Can you work these out from the model? Positions are in its coordinate system, mm. A direction names the side the tool comes from. Round coordinates to 2 decimals unless told otherwise and drop trailing zeros. Loops run counter-clockwise (first coordinate to the right, second up) from the corner with the lowest first, then second, coordinate; pieces in that order, holes last. Notation, with made-up numbers: M 68,84.5 L 114,84.5 A16 ccw 114,92.5 Z; hole C 19.5,-29 d3. An arc over 180 degrees is marked long. Use a Markdown table: item, result. Add a question column.
```python
from build123d import *

# Parameters (mm, degrees)
F3_R        = 44
F3_W        = 60
F3_H        = 60
F4_DEPTH    = 13
F5_T1_DEPTH = 28


# Not quite as in the source:
# - a fillet or chamfer that OpenCascade refuses, or shapes differently, is made with other operations: its cross-section is extruded or revolved along the edge and cut away or added


with BuildPart() as f2:
    # F1 (on Front) → F2 (revolve)
    with BuildSketch(Plane.XZ):
        with BuildLine():
            Line((-18, 6), (0, 6))
            Line((0, 6), (7, 6))
            Line((7, 6), (7, 8))
            Line((7, 8), (9, 8))
            Line((9, 8), (9, 10.5))
            Line((9, 10.5), (19, 10.5))
            Line((19, 10.5), (19, 44))
            Line((19, 44), (6, 44))
            Line((6, 44), (6, 42))
            Line((6, 42), (0, 42))
            Line((0, 42), (0, 20))
            Line((0, 20), (-4, 20))
            ThreePointArc((-4, 20), (-10, 14), (-16, 20))
            Line((-16, 20), (-20, 20))
            Line((-20, 20), (-20, 18))
            Line((-20, 18), (-30, 18))
            Line((-30, 18), (-30, 10.5))
            Line((-30, 10.5), (-20, 10.5))
            Line((-20, 10.5), (-20, 8))
            Line((-20, 8), (-18, 8))
            Line((-18, 8), (-18, 6))
        make_face()
    revolve(axis=Axis((43.6499677598, 0, 0), (1, 0, 0)))

    # F3 (on face) → F4 (cut, through all)
    with BuildSketch(Plane.YZ.offset(19)):
        Circle(F3_R)
        Rectangle(F3_W, F3_H, mode=Mode.SUBTRACT)
    extrude(amount=-F4_DEPTH, mode=Mode.SUBTRACT)

    # F5: fillet of radius 6 on 4 edges, made by hand

    # F5_s2 → F5_t1 (cut)
    with BuildSketch(Plane.YZ.offset(6)):
        with BuildLine():
            ThreePointArc((-30, -24), (-28.2426406871, -28.2426406871), (-24, -30))
            Line((-24, -30), (-30, -30))
            Line((-30, -30), (-30, -24))
        make_face()
        with BuildLine():
            ThreePointArc((24, -30), (28.2426406871, -28.2426406871), (30, -24))
            Line((30, -24), (30, -30))
            Line((30, -30), (24, -30))
        make_face()
        with BuildLine():
            ThreePointArc((-30, 24), (-28.2426406871, 28.2426406871), (-24, 30))
            Line((-24, 30), (-30, 30))
            Line((-30, 30), (-30, 24))
        make_face()
        with BuildLine():
            ThreePointArc((30, 24), (28.2426406871, 28.2426406871), (24, 30))
            Line((24, 30), (30, 30))
            Line((30, 30), (30, 24))
        make_face()
    extrude(amount=F5_T1_DEPTH, mode=Mode.SUBTRACT)


solid = f2.part
```
(1) Suppose I cut it at C-C on y = -21.5. List the corners of the cut face in (x, z) for me, and give its area (3 significant figures).
(2) Suppose I cut it at A-A on x = -1.5. List the corners of the cut face in (y, z) for me, and give its area (3 significant figures).
(3) Suppose I cut it at D-D on z = -34. List the corners of the cut face in (x, y) for me.
(4) Suppose I cut it at B-B on z = 26. List the corners of the cut face in (x, y) for me.
(5) If I drill on probe 1 along Z at (x, y) = (8, 0); probe 2 along Y at (x, z) = (-19, 0), over which ranges is the centre line in solid material (lowest first)? Write a range as [from, to].
(6) On a 3-axis mill with a long thin cutter (end or side, diameter ignored), from which of +Z, -Z, +X, -X, +Y, -Y can I reach the whole of each face in a straight line? I mean faces 5 (the face through (13, -30, 0)), 6 (the face through (6, 3, -31)), 7 (the face through (-18.99, 7.81, -1.73)). Say none if no direction works.
(7) I'm going to push flat-ended pins straight in: pin 1 (6.5 mm diameter, centred on x = 10, y = 12, fed in from +Z); pin 2 (8 mm diameter, centred on y = -30.5, z = 8, fed in from -X); pin 3 (13 mm diameter, centred on y = 0, z = 0, fed in from -X). Where does each tip first touch, or does it pass through?
(8) Thinking about a two-plate mould opening in Z: for faces 1 (the face through (12.409, -28.289, 28.196)), 2 (the face through (9, 8, 2)), 3 (the face through (2.96, -12.62, 40.06)), 4 (the face through (7, -6, 2)), which applies, released by +Z, released by -Z, zero draft, split by the parting line, or undercut?
Results below:
| question | item | result |
|---|---|---|
| 1 | outline | M 0,-36.08 L 6,-36.08 L 6,-30 L 19,-30 L 19,30 L 6,30 L 6,36.08 L 0,36.08 Z |
| 1 | area | 1,210 mm² |
| 2 | outline | C 0,0 d40; hole C 0,0 d12 |
| 2 | area | 1,140 mm² |
| 3 | outline | M 0,-24.66 L 6,-24.66 L 6,24.66 L 0,24.66 Z |
| 4 | outline | M 0,-32.98 L 6,-32.98 L 6,-29.66 L 19,-29.66 L 19,29.66 L 6,29.66 L 6,32.98 L 0,32.98 Z |
| 5 | probe 1 | z = [-30, -8], [8, 30] |
| 5 | probe 2 | y = [-20, -8], [8, 20] |
| 6 | face 5 | +Z, -Z, +X, -Y |
| 6 | face 6 | +X |
| 6 | face 7 | -X |
| 7 | pin 1 | stops at z = 30 |
| 7 | pin 2 | stops at x = 0 |
| 7 | pin 3 | stops at x = -18 |
| 8 | face 1 | released by +Z |
| 8 | face 2 | undercut |
| 8 | face 3 | split by the parting line |
| 8 | face 4 | undercut |
